Source: CAD feature listing. Evaluate the final solid. Frame: model axes, mm. A direction names the side the tool comes from. Coordinates: 2 decimals unless noted, no trailing zeros. Order: outer loops, then holes, each group sorted by start corner. A loop starts at its lowest first (then second) coordinate and runs counter-clockwise, first axis right, second up. Notation, with made-up numbers: (-36, 55) -> (10, 55) arc R21 ccw to (10, 85) -> close; hole circle Ø7 at (84, -39.5). An arc over 180 degrees is marked (long way). Write item = value, one per line. Start each with the question number.
Item 1: Section query D-D (x = -5.5). Output: boundary loops of the cut face in (y, z), then the cut area to 3 significant figures.
Item 2: Section query A-A (x = -0.04). Output: boundary loops of the cut face in (y, z).
Item 3: Contact query for flat-ended pins moving along their axis: pin 1 (6 mm diameter, centred on y = 17, z = 15, fed in from -X); pin 2 (6 mm diameter, centred on y = 12, z = -4, fed in from +X); pin 3 (5 mm diameter, centred on x = 31, y = 13, fed in from +Z); pin 4 (1 mm diameter, centred on x = 10, z = 3.5, fed in from +Y). Output: stop coordinate, or through.
Item 4: Section query B-B (z = -18). Output: boundary loops of the cut face in (x, y).
Item 5: Set-up query: faces 5 (the flat face through (5, 3, 0)), 6 (the cylindrical face through (-0.242, 1.521, 13.463)). Return all of +Z, -Z, +X, -X, +Y, -Y with unobstructed straight access to the full face (end or side cutting, diameter ignored); none if empty.
Item 6: Ray query, line 1 along Z through (x, y) = (-0.04, 1.1); line 2 along X through (y, z) = (2.5, -16); line 3 along X through (y, z) = (2, 0). Return the intervals inside material, ascending. Write a range as [from, to].
Item 7: Section query C-C (z = 15). Output: boundary loops of the cut face in (x, y).
Item 8: Mould query, pull axis Y, two halves, no side actions, for faces 1 (the flat face through (18.2, 2.8, 26.78)), 2 (the flat face through (26.404, 6.698, 0.375)), 3 (the cylindrical face through (37.68, 16.68, -0.37)), 4 (the cylindrical face through (20.77, 0.1, 0.37)). Classes: released by +Y, released by -Y, zero draft, split by the parting line, or undercut.
Autodesk Inventor part; units mm, degrees
ref_plane "YZ Plane" through (0, 0, 0) normal (1, 0, 0) x (0, 1, 0)
ref_plane "XZ Plane" through (0, 0, 0) normal (0, 1, 0) x (-1, 0, 0)
ref_plane "XY Plane" through (0, 0, 0) normal (0, 0, 1) x (1, 0, 0)
sketch "Sketch1" plane through (0, 0, 0) normal (0, 1, 0) x (-1, 0, 0)
  line L0 (10, 26.78) -> (-20, 26.78)
  line L1 (-20, 26.78) -> (-20, -26.78)
  line L2 (-20, -26.78) -> (10, -26.78)
  line L3 (10, -26.78) -> (10, 26.78)
  point P0 (0, 0)
  dimension "d0" = 53.56
  dimension "d1" = 30
  dimension "d2" = 10
  dimension "d3" = 26.78
extrude "Extrusion1" add sketch "Sketch1" along normal blind 3
sketch "Sketch2" plane through (0, 3, 0) normal (0, 1, 0) x (1, 0, 0)
  circle A0 centre (-0.04, 0) radius 1.55
  line L0 (20, -26.78) -> (20, 26.78)
  circle A1 centre (-0.04, -15) radius 1.55
  circle A2 centre (-0.04, 15) radius 1.55
  point P0 (0, 0)
  point P1 (20, 0)
  dimension "d6" = 3.1
  dimension "d7" = 20.04
  dimension "d8" = 0
  dimension "d9" = 3.1
  dimension "d10" = 20.04
  dimension "d11" = 15
  dimension "d12" = 3.1
  dimension "d13" = 20.04
  dimension "d14" = 15
extrude "Extrusion2" cut sketch "Sketch2" against normal blind 3
sketch "Sketch3" plane through (0, 3, 0) normal (0, 1, 0) x (1, 0, 0)
  point P0 (0, 0)
sketch "Sketch4" plane through (20, 0, 26.78) normal (1, 0, 0) x (0, 0, -1)
  line L0 (0, 3) -> (53.56, 3)
  line L1 (53.56, 3) -> (53.56, 0)
  line L2 (53.56, 0) -> (0, 0)
  line L3 (0, 0) -> (0, 3)
  line L4 (0, 3) -> (53.56, 3)
  line L5 (0, 0) -> (0, 3)
  point P0 (26.78, 0)
  dimension "d17" = 3
  dimension "d18" = 53.56
  dimension "d19" = 0
  dimension "d20" = 0
revolve "Revolution2" add sketch "Sketch4" angle 30 about axis through (20, 3, 26.78) along (0, 0, 1)
sketch "Sketch6" plane through (20, 3, 26.78) normal (0.8660254, 0.5, 0) x (0, 0, -1)
  line L0 (0, 0) -> (53.56, 0)
  line L1 (53.56, 0) -> (53.56, -3)
  line L2 (53.56, -3) -> (0, -3)
  line L3 (0, -3) -> (0, 0)
  line L4 (0, 0) -> (53.56, 0)
  line L5 (0, 0) -> (0, -3)
  point P0 (26.78, 7.4019)
  dimension "d26" = 53.56
  dimension "d27" = 3
  dimension "d28" = 0
  dimension "d29" = 0
extrude "Extrusion3" add sketch "Sketch6" along normal blind 15
sketch "Sketch7" plane through (32.9904, 10.5, 26.78) normal (0.8660254, 0.5, 0) x (0, 0, -1)
  line L0 (0, 0) -> (53.56, 0)
  line L1 (53.56, 0) -> (53.56, -3)
  line L2 (53.56, -3) -> (0, -3)
  line L3 (0, -3) -> (0, 0)
  line L4 (0, -3) -> (53.56, -3)
  line L5 (0, 0) -> (0, -3)
  point P0 (26.78, 7.4019)
  dimension "d32" = 53.56
  dimension "d33" = 3
  dimension "d34" = 0
  dimension "d35" = 0
sketch "Sketch8" plane through (32.9904, 10.5, 26.78) normal (0.8660254, 0.5, 0) x (0, 0, -1)
  line L0 (-5.6464, 10) -> (58.6102, 10)
  line L1 (58.6102, 10) -> (58.6102, -7.2897)
  line L2 (58.6102, -7.2897) -> (-5.6464, -7.2897)
  line L3 (-5.6464, -7.2897) -> (-5.6464, 10)
  line L4 (53.56, 0) -> (0, 0)
  line L5 (53.56, -3) -> (53.56, 0)
  point P0 (26.78, 7.4019)
  dimension "d38" = 64.2566
  dimension "d39" = 17.2897
  dimension "d40" = 10
  dimension "d41" = 5.0502
revolve "Revolution4" add sketch "Sketch7" angle 90 about axis through (27.9904, 19.1603, 32.4264) along (0, 0, 1)
properties part number "gripper_frame"
Computed:
q1.outline = (0, -26.78) -> (3, -26.78) -> (3, 26.78) -> (0, 26.78) -> close
q1.area = 161 mm^2
q2.outline = (0, -26.78) -> (3, -26.78) -> (3, -16.55) -> (0, -16.55) -> close; (0, -13.45) -> (3, -13.45) -> (3, -1.55) -> (0, -1.55) -> close; (0, 1.55) -> (3, 1.55) -> (3, 13.45) -> (0, 13.45) -> close; (0, 16.55) -> (3, 16.55) -> (3, 26.78) -> (0, 26.78) -> close
q3.pin_1 = 36.56
q3.pin_2 = 40.31
q3.pin_3 = through
q3.pin_4 = 3
q4.outline = (-10, 0) -> (20, 0) arc R3 ccw to (21.5, 0.4) -> (34.49, 7.9) arc R13 ccw to (39.25, 25.66) -> (36.65, 24.16) arc R10 cw to (32.99, 10.5) -> (20, 3) -> (-10, 3) -> close
q5.face_5 = +Z, -Z, -X, +Y
q5.face_6 = +Y, -Y
q6.line_1 = [-26.78, -16.55], [-13.45, -1.55], [1.55, 13.45], [16.55, 26.78]
q6.line_2 = [-10, -1.22], [1.14, 25.13]
q6.line_3 = [-10, -1.59], [1.51, 24.27]
q7.outline = (-10, 0) -> (-1.59, 0) -> (-1.59, 3) -> (-10, 3) -> close; (1.51, 0) -> (20, 0) arc R3 ccw to (21.5, 0.4) -> (34.49, 7.9) arc R13 ccw to (39.25, 25.66) -> (36.65, 24.16) arc R10 cw to (32.99, 10.5) -> (20, 3) -> (1.51, 3) -> close
q8.face_1 = zero draft
q8.face_2 = released by +Y
q8.face_3 = undercut
q8.face_4 = released by -Y
